Source: CAD feature listing. Evaluate the final solid. Frame: model axes, mm. A direction names the side the tool comes from. Coordinates: 2 decimals unless noted, no trailing zeros. Loops run counter-clockwise (first coordinate to the right, second up) from the corner with the lowest first, then second, coordinate; pieces in that order, holes last.
Item 1: Pin query (flat end, axial travel): pin 1 Ø2 at (x, y) = (66, 0) entering from -Z; pin 2 Ø1.5 at (x, z) = (77.5, -1.5) entering from +Y; pin 3 Ø3 at (x, y) = (45.5, 0) entering from +Z. Return the tip coordinate at first contact, or that it passes through.
Item 2: Section query A-A, the plane x = 6. Return the cut outline in (y, z).
Item 3: Pull-direction query (Y, two-part tool) for faces 1 (the flat face through (17, 1.5, -1)), 2 (the flat face through (37, 4, -1)), 3 (the cylindrical face through (-4, 0, -1)), 4 (the flat face through (62, -1.5, -1)); classes: +Y half, -Y half, draft (parallel to the pull), parting line (faces both ways), or undercut.
Item 4: Section query B-B, the plane x = 32. Return the cut outline in (y, z).
Item 5: Section query C-C, the plane y = 0. State how many separate pieces and enclosed holes the cut face has, then the cut area to 3 significant figures.
Item 6: Reachability of faces 5 (the flat face through (77, -1.5, -1)), 6 (the flat face through (22, 0, -0.8)), 7 (the flat face through (67, 0, -2.2)) from +Z, -Z, +X, -X, +Y, -Y: full face, straight path, thin tool, end or side. Return the list, or none.
Item 7: Line query: probe 1 along Y at (x, z) = (75, -1); probe 2 along Z at (x, y) = (61.5, 2.75); probe 3 along Y at (x, z) = (45.5, -1.9). Output: solid intervals per line, ascending.
```python
from build123d import *

# Parameters (mm, degrees)
EXTRUDE_1_DEPTH          = 3
CUT_EXTRUDE_1_REACH      = 81.158
SKETCH_3_R               = 3.25
CUT_EXTRUDE_2_DEPTH      = 0.8
CUT_EXTRUDE_START        = -2.2
SKETCH_3_2_R             = 3.25
CUT_EXTRUDE_3_DEPTH      = 0.8
CUT_EXTRUDE_4_DEPTH      = 0.8
SKETCH_5_W               = 7
SKETCH_5_H               = 4
CUT_EXTRUDE_6_DEPTH      = 0.8
MIRROR_8_COPY_1_REACH    = 81.158
MIRROR_8_COPY_2_SKETCH_R = 3.25
MIRROR_8_COPY_2_DEPTH    = 0.8
MIRROR_START             = -2.2
MIRROR_8_COPY_3_SKETCH_R = 3.25
MIRROR_8_COPY_3_DEPTH    = 0.8
MIRROR_8_COPY_4_DEPTH    = 0.8
MIRROR_8_COPY_5_SKETCH_W = 7
MIRROR_8_COPY_5_SKETCH_H = 4
MIRROR_8_COPY_5_DEPTH    = 0.8
MIRROR_8_COPY_6_REACH    = 81.158
MIRROR_8_COPY_7_SKETCH_R = 3.25
MIRROR_8_COPY_7_DEPTH    = 0.8
MIRROR_8_COPY_8_SKETCH_R = 3.25
MIRROR_8_COPY_8_DEPTH    = 0.8


with BuildPart() as part:
    # 草图1 → 凸台-拉伸1 (new body)
    with BuildSketch(Plane.XY):
        with BuildLine():
            Line((0, 4), (75, 4))
            ThreePointArc((75, 4), (79, 0), (75, -4))
            Line((75, -4), (0, -4))
            ThreePointArc((0, -4), (-4, 0), (0, 4))
        make_face()
    extrude(amount=-EXTRUDE_1_DEPTH)

    # 草图2 → 切除-拉伸1 (cut, up to next)
    with BuildSketch(Plane.XY, mode=Mode.PRIVATE) as cut_extrude_1_sk1:
        with BuildLine():
            Line((1.322875656, -1.5), (2.883140649, -1.5))
            ThreePointArc((2.883140649, -1.5), (3.25, 0), (2.883140649, 1.5))
            Line((2.883140649, 1.5), (1.322875656, 1.5))
            ThreePointArc((1.322875656, 1.5), (0, 2), (-1.322875656, 1.5))
            Line((-1.322875656, 1.5), (-2.883140649, 1.5))
            ThreePointArc((-2.883140649, 1.5), (-3.25, 0), (-2.883140649, -1.5))
            Line((-2.883140649, -1.5), (-1.322875656, -1.5))
            ThreePointArc((-1.322875656, -1.5), (0, -2), (1.322875656, -1.5))
        make_face()
    cut_extrude_1_tool1 = extrude(cut_extrude_1_sk1.sketch, amount=-CUT_EXTRUDE_1_REACH, mode=Mode.PRIVATE) & part.part
    cut_extrude_1 = cut_extrude_1_tool1.solids().sort_by_distance((0, 0, 0))[0]
    add(cut_extrude_1, mode=Mode.SUBTRACT)

    # 草图3 → 切除-拉伸2 (cut)
    with BuildSketch(Plane.XY):
        Circle(SKETCH_3_R)
    cut_extrude_2 = extrude(amount=-CUT_EXTRUDE_2_DEPTH, mode=Mode.SUBTRACT)

    # 草图3<2> → 切除-拉伸3 (cut)
    with BuildSketch(Plane.XY.offset(CUT_EXTRUDE_START)):
        Circle(SKETCH_3_2_R)
    cut_extrude_3 = extrude(amount=-CUT_EXTRUDE_3_DEPTH, mode=Mode.SUBTRACT)

    # 草图4 → 切除-拉伸4 (cut)
    with BuildSketch(Plane.XY):
        with BuildLine():
            Line((3.464101615, 2), (11.535898385, 2))
            ThreePointArc((11.535898385, 2), (11, 0), (11.535898385, -2))
            Line((11.535898385, -2), (3.464101615, -2))
            ThreePointArc((3.464101615, -2), (4, 0), (3.464101615, 2))
        make_face()
    cut_extrude_4 = extrude(amount=-CUT_EXTRUDE_4_DEPTH, mode=Mode.SUBTRACT)

    # 草图5 → 切除-拉伸6 (cut)
    with BuildSketch(Plane(origin=(0, 0, -3), x_dir=(-1, 0, 0), z_dir=(0, 0, -1))):
        with Locations((-7.5, 0)):
            Rectangle(SKETCH_5_W, SKETCH_5_H)
    cut_extrude_6 = extrude(amount=-CUT_EXTRUDE_6_DEPTH, mode=Mode.SUBTRACT)

    # 镜向1: 切除-拉伸1, 切除-拉伸2, 切除-拉伸3 across plane
    add(cut_extrude_1.mirror(Plane(origin=(7.5, 0, 0), x_dir=(0, 0, 1), z_dir=(1, 0, 0))), mode=Mode.SUBTRACT)
    add(cut_extrude_2.mirror(Plane(origin=(7.5, 0, 0), x_dir=(0, 0, 1), z_dir=(1, 0, 0))), mode=Mode.SUBTRACT)
    add(cut_extrude_3.mirror(Plane(origin=(7.5, 0, 0), x_dir=(0, 0, 1), z_dir=(1, 0, 0))), mode=Mode.SUBTRACT)

    # 镜向3: 切除-拉伸4, 切除-拉伸6 across plane
    add(cut_extrude_4.mirror(Plane(origin=(15, 0, 0), x_dir=(0, 0, 1), z_dir=(1, 0, 0))), mode=Mode.SUBTRACT)
    add(cut_extrude_6.mirror(Plane(origin=(15, 0, 0), x_dir=(0, 0, 1), z_dir=(1, 0, 0))), mode=Mode.SUBTRACT)

    # 镜向4: 切除-拉伸4, 切除-拉伸6 across plane
    add(cut_extrude_4.mirror(Plane(origin=(22.5, 0, 0), x_dir=(0, 0, 1), z_dir=(1, 0, 0))), mode=Mode.SUBTRACT)
    add(cut_extrude_6.mirror(Plane(origin=(22.5, 0, 0), x_dir=(0, 0, 1), z_dir=(1, 0, 0))), mode=Mode.SUBTRACT)

    # 镜向7: 切除-拉伸1, 切除-拉伸2, 切除-拉伸3 across plane
    add(cut_extrude_1.mirror(Plane(origin=(15, 0, 0), x_dir=(0, 0, 1), z_dir=(1, 0, 0))), mode=Mode.SUBTRACT)
    add(cut_extrude_2.mirror(Plane(origin=(15, 0, 0), x_dir=(0, 0, 1), z_dir=(1, 0, 0))), mode=Mode.SUBTRACT)
    add(cut_extrude_3.mirror(Plane(origin=(15, 0, 0), x_dir=(0, 0, 1), z_dir=(1, 0, 0))), mode=Mode.SUBTRACT)

    # 镜向8: 切除-拉伸1, 切除-拉伸2, 切除-拉伸3, 切除-拉伸4, 切除-拉伸6 across plane
    add(cut_extrude_1.mirror(Plane(origin=(37.5, 0, 0), x_dir=(0, 0, 1), z_dir=(1, 0, 0))), mode=Mode.SUBTRACT)
    add(cut_extrude_2.mirror(Plane(origin=(37.5, 0, 0), x_dir=(0, 0, 1), z_dir=(1, 0, 0))), mode=Mode.SUBTRACT)
    add(cut_extrude_3.mirror(Plane(origin=(37.5, 0, 0), x_dir=(0, 0, 1), z_dir=(1, 0, 0))), mode=Mode.SUBTRACT)
    add(cut_extrude_4.mirror(Plane(origin=(37.5, 0, 0), x_dir=(0, 0, 1), z_dir=(1, 0, 0))), mode=Mode.SUBTRACT)
    add(cut_extrude_6.mirror(Plane(origin=(37.5, 0, 0), x_dir=(0, 0, 1), z_dir=(1, 0, 0))), mode=Mode.SUBTRACT)

    # 镜向8 copy 1 sketch → 镜向8 copy 1 (cut, up to next)
    with BuildSketch(Plane(origin=(60, 0, 0), x_dir=(1, 0, 0), z_dir=(0, 0, 1)), mode=Mode.PRIVATE) as mirror_8_copy_1_sk1:
        with BuildLine():
            Line((1.322875656, -1.5), (2.883140649, -1.5))
            ThreePointArc((2.883140649, -1.5), (3.25, 0), (2.883140649, 1.5))
            Line((2.883140649, 1.5), (1.322875656, 1.5))
            ThreePointArc((1.322875656, 1.5), (0, 2), (-1.322875656, 1.5))
            Line((-1.322875656, 1.5), (-2.883140649, 1.5))
            ThreePointArc((-2.883140649, 1.5), (-3.25, 0), (-2.883140649, -1.5))
            Line((-2.883140649, -1.5), (-1.322875656, -1.5))
            ThreePointArc((-1.322875656, -1.5), (0, -2), (1.322875656, -1.5))
        make_face()
    mirror_8_copy_1_tool1 = extrude(mirror_8_copy_1_sk1.sketch, amount=-MIRROR_8_COPY_1_REACH, mode=Mode.PRIVATE) & part.part
    add(mirror_8_copy_1_tool1.solids().sort_by_distance((60, 0, 0))[0], mode=Mode.SUBTRACT)

    # 镜向8 copy 2 sketch → 镜向8 copy 2 (cut)
    with BuildSketch(Plane(origin=(60, 0, 0), x_dir=(1, 0, 0), z_dir=(0, 0, 1))):
        Circle(MIRROR_8_COPY_2_SKETCH_R)
    extrude(amount=-MIRROR_8_COPY_2_DEPTH, mode=Mode.SUBTRACT)

    # 镜向8 copy 3 sketch → 镜向8 copy 3 (cut)
    with BuildSketch(Plane(origin=(60, 0, 0), x_dir=(1, 0, 0), z_dir=(0, 0, 1)).offset(MIRROR_START)):
        Circle(MIRROR_8_COPY_3_SKETCH_R)
    extrude(amount=-MIRROR_8_COPY_3_DEPTH, mode=Mode.SUBTRACT)

    # 镜向8 copy 4 sketch → 镜向8 copy 4 (cut)
    with BuildSketch(Plane(origin=(45, 0, 0), x_dir=(1, 0, 0), z_dir=(0, 0, 1))):
        with BuildLine():
            Line((3.464101615, 2), (11.535898385, 2))
            ThreePointArc((11.535898385, 2), (11, 0), (11.535898385, -2))
            Line((11.535898385, -2), (3.464101615, -2))
            ThreePointArc((3.464101615, -2), (4, 0), (3.464101615, 2))
        make_face()
    extrude(amount=-MIRROR_8_COPY_4_DEPTH, mode=Mode.SUBTRACT)

    # 镜向8 copy 5 sketch → 镜向8 copy 5 (cut)
    with BuildSketch(Plane(origin=(45, 0, -3), x_dir=(-1, 0, 0), z_dir=(0, 0, -1))):
        with Locations((-7.5, 0)):
            Rectangle(MIRROR_8_COPY_5_SKETCH_W, MIRROR_8_COPY_5_SKETCH_H)
    extrude(amount=-MIRROR_8_COPY_5_DEPTH, mode=Mode.SUBTRACT)

    # 镜向8 copy 6 sketch → 镜向8 copy 6 (cut, up to next)
    with BuildSketch(Plane(origin=(45, 0, 0), x_dir=(1, 0, 0), z_dir=(0, 0, 1)), mode=Mode.PRIVATE) as mirror_8_copy_6_sk1:
        with BuildLine():
            Line((1.322875656, -1.5), (2.883140649, -1.5))
            ThreePointArc((2.883140649, -1.5), (3.25, 0), (2.883140649, 1.5))
            Line((2.883140649, 1.5), (1.322875656, 1.5))
            ThreePointArc((1.322875656, 1.5), (0, 2), (-1.322875656, 1.5))
            Line((-1.322875656, 1.5), (-2.883140649, 1.5))
            ThreePointArc((-2.883140649, 1.5), (-3.25, 0), (-2.883140649, -1.5))
            Line((-2.883140649, -1.5), (-1.322875656, -1.5))
            ThreePointArc((-1.322875656, -1.5), (0, -2), (1.322875656, -1.5))
        make_face()
    mirror_8_copy_6_tool1 = extrude(mirror_8_copy_6_sk1.sketch, amount=-MIRROR_8_COPY_6_REACH, mode=Mode.PRIVATE) & part.part
    add(mirror_8_copy_6_tool1.solids().sort_by_distance((45, 0, 0))[0], mode=Mode.SUBTRACT)

    # 镜向8 copy 7 sketch → 镜向8 copy 7 (cut)
    with BuildSketch(Plane(origin=(45, 0, 0), x_dir=(1, 0, 0), z_dir=(0, 0, 1))):
        Circle(MIRROR_8_COPY_7_SKETCH_R)
    extrude(amount=-MIRROR_8_COPY_7_DEPTH, mode=Mode.SUBTRACT)

    # 镜向8 copy 8 sketch → 镜向8 copy 8 (cut)
    with BuildSketch(Plane(origin=(45, 0, 0), x_dir=(1, 0, 0), z_dir=(0, 0, 1)).offset(MIRROR_START)):
        Circle(MIRROR_8_COPY_8_SKETCH_R)
    extrude(amount=-MIRROR_8_COPY_8_DEPTH, mode=Mode.SUBTRACT)


solid = part.part
```
Verdict:
1. pin 1: stops at z = -2.2
1. pin 2: stops at y = 3.6
1. pin 3: passes through
2. outline: (-4, -3) - (-2, -3) - (-2, -2.2) - (2, -2.2) - (2, -3) - (4, -3) - (4, 0) - (2, 0) - (2, -0.8) - (-2, -0.8) - (-2, 0) - (-4, 0) - close
3. face 1: undercut
3. face 2: +Y half
3. face 3: parting line
3. face 4: undercut
4. outline: (-4, -3) - (-2.56, -3) - (-2.56, -2.2) - (-1.5, -2.2) - (-1.5, -0.8) - (-2.56, -0.8) - (-2.56, 0) - (-4, 0) - close; (1.5, -2.2) - (2.56, -2.2) - (2.56, -3) - (4, -3) - (4, 0) - (2.56, 0) - (2.56, -0.8) - (1.5, -0.8) - close
5. separate pieces: 7
5. enclosed holes: 0
5. area: 76.0 mm2
6. face 5: +Z, -Z
6. face 6: +Z
6. face 7: -Z
7. probe 1: y = -4 to -2, 2 to 4
7. probe 2: z = -2.2 to -0.8
7. probe 3: y = -4 to -1.94, 1.94 to 4
